The listing builds one solid part. Answer for the finished solid, in the listing's coordinates (mm). A direction names the side the tool comes from. Give positions to 0.01 mm unless a question says otherwise; leave off trailing zeros. Write each loop counter-clockwise with the first axis right and the second up, starting at its lowest first coordinate (ties: lowest second). Pieces come first, ordered by that corner, then holes. Notation, with made-up numbers: (-34.75, 68.5) - (20.25, 68.5) arc R22 cw to (20.25, 74.5) - close; hole circle Ø1 at (-7.75, 24.25). An arc over 180 degrees is marked (long way). Answer as CSV lines item,"result". Start each with the question number.
(1) Find section D-D (z = 14). Write down the section's boundary in (x, y), then the cut area to 3 significant figures.
(2) Find section A-A (z = 0). Write down the section's boundary in (x, y) (3 decimals).
(3) Find section C-C (z = 8.5). Write down the section's boundary in (x, y), then the cut area to 3 significant figures.
(4) Each of these flat-tipped pins is pushed along its axis until it touches: pin 1 Ø3.5 at (x, y) = (6.5, 5) entering from +Z; pin 2 Ø6 at (y, z) = (3.5, 9.5) entering from +X; pin 3 Ø5 at (y, z) = (-0.5, 12) entering from -X. Where does it stop, or does it pass through?
(5) Find section B-B (x = 32). Write down the section's boundary in (y, z), then the cut area to 3 significant figures.
(6) For faces 4 (the face through (28, 6, 0)), 5 (the face through (7, 5, -0.59)), 6 (the face through (12.77, 1.01, 2.21)), determine the directions among +Z, -Z, +X, -X, +Y, -Y from which every point of the face is accessible in a straight line to the end or side of a thin tool.
(7) For a pull along Y with two mould halves and no side action, classify faces 1 (the face through (9.57, 5.248, 0.995)), 2 (the face through (12.12, -2, 0)), 3 (the face through (35.5, 3, -2)) as pulls with the +Y half, pulls with the -Y half, needs draft (parallel to the pull), parting line crosses it, or undercut.
(8) Straight lines are drawn through the part: probe 1 along Y at (x, z) = (0, 9); probe 2 along Z at (x, y) = (18, 4.5); probe 3 along X at (y, z) = (1.5, 4). For each, find the intervals that lie inside material, in ascending order.
from build123d import *

# Parameters (mm, degrees)
BOSS_EXTRUDE3_DEPTH  = 3
SKETCH2_R            = 2.9999999999999982
BOSS_EXTRUDE4_DEPTH  = 16.205
SKETCH5_R            = 1.96
CUT_EXTRUDE2_DEPTH   = 32.80000000000002
SKETCH6_R            = 1.465
BOSS_EXTRUDE7_DEPTH  = 3
FILLET1_R            = 0.5
BOSS_EXTRUDE8_DEPTH  = 0.59
BOSS_EXTRUDE9_DEPTH  = 13.35
FILLET7_R            = 0.5
FILLET8_R            = 0.5
BOSS_EXTRUDE10_DEPTH = 3
CUT_EXTRUDE4_DEPTH   = 3
BOSS_EXTRUDE11_DEPTH = 0.59
BOSS_EXTRUDE12_DEPTH = 1.395
CUT_EXTRUDE6_DEPTH   = 20.895000000000014
CUT_EXTRUDE7_DEPTH   = 0.25
CUT_EXTRUDE8_DEPTH   = 0.25
FILLET9_R            = 0.5
FILLET10_R           = 0.5
CUT_EXTRUDE9_DEPTH   = 2.5
CUT_EXTRUDE10_DEPTH  = 2.5
CUT_EXTRUDE12_DEPTH  = 2.5
CUT_EXTRUDE14_START  = -2.5
CUT_EXTRUDE14_DEPTH  = 2.5


with BuildPart() as part:
    # Sketch1 → Boss-Extrude3 (new, symmetric)
    with BuildSketch(Plane.XY):
        with BuildLine():
            ThreePointArc((2.9999999999999982, 2.9999999999999973), (2.1213203435596406, 0.8786796564403563), (-5.5e-16, 0))
            Line((0, 0), (36.5, 0))
            Line((36.5, 0), (36.5, 6))
            Line((36.5, 6), (20.749999999999996, 5.999999999999999))
            ThreePointArc((20.749999999999996, 5.999999999999999), (20.435386233554034, 4.445031090493969), (19.54103584523481, 3.134669493650969))
            ThreePointArc((19.54103584523481, 3.1346694936509705), (17.593985916344508, 2.2872332130112563), (15.573673818645423, 2.9410609450836516))
            Line((15.573673818645423, 2.9410609450836516), (11.749999999999998, 5.9999999999999964))
            Line((11.749999999999998, 5.9999999999999964), (0, 5.9999999999999964))
            ThreePointArc((1.8e-16, 5.9999999999999964), (2.1213203435596415, 5.121320343559639), (2.9999999999999982, 2.9999999999999982))
        make_face()
    extrude(amount=BOSS_EXTRUDE3_DEPTH, both=True)

    # Sketch2 → Boss-Extrude4 (add, symmetric)
    with BuildSketch(Plane.XY):
        with Locations((0, 2.9999999999999982)):
            Circle(SKETCH2_R)
    extrude(amount=BOSS_EXTRUDE4_DEPTH, both=True)

    # Sketch5 → Cut-Extrude2 (cut)
    with BuildSketch(Plane.XY.offset(16.205)):
        with Locations((0, 2.9999999999999982)):
            Circle(SKETCH5_R)
    extrude(amount=-CUT_EXTRUDE2_DEPTH, mode=Mode.SUBTRACT)

    # Sketch6 → Boss-Extrude7 (add)
    with BuildSketch(Plane(origin=(36.5, 0, 0), x_dir=(0, 0, -1), z_dir=(1, 0, 0))):
        with Locations((0, 2.999999999999999)):
            Circle(SKETCH6_R)
    extrude(amount=BOSS_EXTRUDE7_DEPTH)

    # Fillet1
    fillet1_edges = [part.edges().sort_by_distance(p)[0] for p in [
        (39.5, 2.9999999999999987, 1.465),
    ]]
    fillet(fillet1_edges, radius=FILLET1_R)

    # Sketch12 → Boss-Extrude8 (add, symmetric)
    with BuildSketch(Plane.XY):
        with BuildLine():
            Line((12.12, -2.99e-15), (12.12, -3.970000000000003))
            Line((12.12, -3.970000000000003), (10.479512267647207, -5.6104877323527935))
            Line((10.479512267647207, -5.6104877323527935), (1.2595122676472073, -5.610487732352795))
            Line((1.2595122676472073, -5.610487732352795), (-2.8063517241754403, -1.5446237405301462))
            Line((-2.8063517241754403, -1.5446237405301462), (-2.8063517241754403, 1.939627423865778))
            ThreePointArc((-2.8063517241754403, 1.939627423865778), (-1.7057083970593148, 0.5320942351456543), (0, 0))
            Line((0, 0), (12.12, -2.99e-15))
        make_face()
    extrude(amount=BOSS_EXTRUDE8_DEPTH, both=True)

    # Sketch14 → Boss-Extrude9 (add, symmetric)
    with BuildSketch(Plane.XY):
        with BuildLine():
            Line((3.9999999999999982, 2.4999999999999982), (3.9999999999999982, 3.4999999999999982))
            Line((3.9999999999999982, 3.4999999999999982), (2.9580398915498067, 3.4999999999999982))
            ThreePointArc((2.9580398915498067, 3.4999999999999982), (2.999999999999999, 2.9999999999999982), (2.9580398915498067, 2.4999999999999982))
            Line((2.9580398915498067, 2.4999999999999982), (3.9999999999999982, 2.4999999999999982))
        make_face()
    extrude(amount=BOSS_EXTRUDE9_DEPTH, both=True)

    # Fillet7
    fillet7_edges = [part.edges().sort_by_distance(p)[0] for p in [
        (3.9999999999999982, 2.9999999999999982, 13.35),
    ]]
    fillet(fillet7_edges, radius=FILLET7_R)

    # Fillet8
    fillet8_edges = [part.edges().sort_by_distance(p)[0] for p in [
        (3.9999999999999982, 2.9999999999999982, -13.35),
    ]]
    fillet(fillet8_edges, radius=FILLET8_R)

    # Sketch15 → Boss-Extrude10 (add, symmetric)
    with BuildSketch(Plane.XY):
        Polygon((5.875, 5.9999999999999964), (27.07720850874597, 5.999999999999999), (27.07720850874597, 1.48970114733157), (5.875, 1.48970114733157), align=None)
    extrude(amount=BOSS_EXTRUDE10_DEPTH, both=True)

    # Sketch16 → Cut-Extrude4 (cut, symmetric)
    with BuildSketch(Plane.XY):
        with BuildLine():
            ThreePointArc((13.27019347571673, 1.2228284271177183), (12.760871493283885, 1.00722209344764), (12.214852275986694, 1.0953015306060352))
            Line((12.214852275986694, 1.0953015306060352), (1.8, 6))
            Line((1.8, 6), (19.169999999999998, 6.000000000000002))
            Line((19.169999999999998, 6.000000000000002), (13.27019347571673, 1.2228284271177183))
        make_face()
    extrude(amount=CUT_EXTRUDE4_DEPTH, both=True, mode=Mode.SUBTRACT)

    # Sketch17 → Boss-Extrude11 (add, symmetric)
    with BuildSketch(Plane.XY):
        Polygon((1.8, 6), (19.169999999999998, 5.999999999999999), (19.169999999999998, 0.49690997030879536), (1.8, 0.49690997030879536), (4.890483943976141, 2.396162656787146), align=None)
    extrude(amount=BOSS_EXTRUDE11_DEPTH, both=True)

    # Sketch19 → Boss-Extrude12 (add, symmetric)
    with BuildSketch(Plane.XY):
        with BuildLine():
            Line((8.17, 3.000156274700533), (10.684653005804094, 7.569117176028711))
            ThreePointArc((10.684653005804094, 7.569117176028711), (12.655773390851454, 8.734228825048191), (14.626946759842125, 7.569206818212221))
            Line((14.626946759842125, 7.569206818212221), (15.490695774172368, 5.999999999999999))
            Line((15.490695774172368, 5.999999999999999), (16.624997623308392, 3.9392692019970994))
            Line((16.624997623308392, 3.9392692019970994), (13.27019347571673, 1.2228284271177192))
            ThreePointArc((13.27019347571673, 1.2228284271177192), (12.760871493283883, 1.0072220934476446), (12.21485227598669, 1.0953015306060374))
            Line((12.21485227598669, 1.0953015306060374), (8.17, 3.000156274700533))
        make_face()
    extrude(amount=BOSS_EXTRUDE12_DEPTH, both=True)

    # Sketch20 → Cut-Extrude6 (cut, symmetric)
    with BuildSketch(Plane.XY.offset(1.395)):
        with BuildLine():
            ThreePointArc((14.155824552668768, 6.484228825629862), (12.655824552668768, 7.984228825629863), (11.155824552668768, 6.484228825629862))
            ThreePointArc((11.15582455266877, 6.484228825629865), (12.655824552668765, 4.984228825629861), (14.155824552668767, 6.484228825629859))
        make_face()
    extrude(amount=CUT_EXTRUDE6_DEPTH, both=True, mode=Mode.SUBTRACT)

    # Sketch21 → Cut-Extrude7 (cut, symmetric)
    with BuildSketch(Plane.XY.offset(1.395)):
        with BuildLine():
            Line((11.155824552668768, 6.484228825629862), (9.018377782257767, 2.60062711193924))
            Line((9.018377782257767, 2.60062711193924), (8.17, 3.000156274700535))
            Line((8.17, 3.000156274700535), (10.684653005804092, 7.569117176028711))
            ThreePointArc((10.684653005804092, 7.569117176028711), (12.655773390851452, 8.734228825048183), (14.626946759842125, 7.569206818212221))
            Line((14.626946759842125, 7.569206818212221), (16.62499762330839, 3.9392692019970985))
            Line((16.62499762330839, 3.9392692019970985), (15.886023032964967, 3.3409091724705715))
            Line((15.886023032964967, 3.3409091724705715), (14.155824552668767, 6.484228825629862))
            ThreePointArc((14.155824552668767, 6.484228825629862), (12.655824552668768, 4.984228825629862), (11.155824552668768, 6.484228825629862))
        make_face()
    extrude(amount=CUT_EXTRUDE7_DEPTH, both=True, mode=Mode.SUBTRACT)

    # Sketch22 → Cut-Extrude8 (cut, symmetric)
    with BuildSketch(Plane(origin=(0, 0, -1.395), x_dir=(-1, 0, 0), z_dir=(0, 0, -1))):
        with BuildLine():
            Line((-14.155824552668767, 6.484228825629862), (-15.886023032964967, 3.340909172470571))
            Line((-15.886023032964967, 3.340909172470571), (-16.624997623308392, 3.9392692019971034))
            Line((-16.624997623308392, 3.9392692019971034), (-14.626946759842125, 7.569206818212221))
            ThreePointArc((-14.626946759842125, 7.569206818212221), (-12.655773390851454, 8.73422882504819), (-10.684653005804092, 7.569117176028711))
            Line((-10.684653005804092, 7.569117176028711), (-8.17, 3.000156274700535))
            Line((-8.17, 3.000156274700535), (-9.018377782257769, 2.600627111939241))
            Line((-9.018377782257769, 2.600627111939241), (-11.155824552668768, 6.484228825629862))
            ThreePointArc((-11.155824552668768, 6.484228825629862), (-12.655824552668768, 4.984228825629864), (-14.155824552668767, 6.484228825629862))
        make_face()
    extrude(amount=CUT_EXTRUDE8_DEPTH, both=True, mode=Mode.SUBTRACT)

    # Fillet9
    fillet9_edges = [part.edges().sort_by_distance(p)[0] for p in [
        (15.625972191575258, 5.754238010104662, -1.145),
        (12.655773390851452, 8.73422882504819, -1.145),
        (9.427326502902046, 5.2846367253646225, -1.145),
    ]]
    fillet(fillet9_edges, radius=FILLET9_R)

    # Fillet10
    fillet10_edges = [part.edges().sort_by_distance(p)[0] for p in [
        (9.427326502902046, 5.2846367253646225, 1.145),
        (12.655773390851452, 8.734228825048183, 1.145),
        (15.625972191575258, 5.754238010104659, 1.145),
    ]]
    fillet(fillet10_edges, radius=FILLET10_R)

    # Sketch23 → Cut-Extrude9 (cut)
    with BuildSketch(Plane(origin=(0, 0, -3), x_dir=(-1, 0, 0), z_dir=(0, 0, -1))):
        Polygon((-35.5, 5), (-35.5, 1), (-14.230000308321648, 1), (-19.169999999999998, 5), align=None)
    extrude(amount=-CUT_EXTRUDE9_DEPTH, mode=Mode.SUBTRACT)

    # Sketch24 → Cut-Extrude10 (cut)
    with BuildSketch(Plane(origin=(0, 0, -3), x_dir=(-1, 0, 0), z_dir=(0, 0, -1))):
        with BuildLine():
            Line((-10.07009080824153, 1), (-3.4641016151377535, 1))
            ThreePointArc((-3.4641016151377535, 1), (-3.9566645904895195, 2.412798741174382), (-3.895636139676663, 3.9077549599121406))
            Line((-3.895636139676663, 3.9077549599121406), (-10.07009080824153, 1))
        make_face()
    extrude(amount=-CUT_EXTRUDE10_DEPTH, mode=Mode.SUBTRACT)

    # Sketch25 → Cut-Extrude12 (cut)
    with BuildSketch(Plane.XY.offset(3)):
        Polygon((19.524095671942906, 5), (35.5, 5), (35.5, 1), (14.584095980264548, 0.9999999999999983), align=None)
    extrude(amount=-CUT_EXTRUDE12_DEPTH, mode=Mode.SUBTRACT)

    # Sketch26 → Cut-Extrude14 (cut)
    with BuildSketch(Plane.XY.offset(3).offset(CUT_EXTRUDE14_START)):
        with BuildLine():
            Line((3.4641016151377535, 1), (10.070090808241538, 1))
            Line((10.070090808241538, 1), (3.8956361396766637, 3.9077549599121406))
            ThreePointArc((3.8956361396766637, 3.9077549599121406), (3.956664590489521, 2.4127987411743836), (3.4641016151377535, 1))
        make_face()
    extrude(amount=CUT_EXTRUDE14_DEPTH, mode=Mode.SUBTRACT)


solid = part.part
Result set:
1,outline,"circle Ø6 at (0, 3); hole circle Ø3.92 at (0, 3)"
1,area,"16.2 mm^2"
2,outline,"(-2.806, -1.545) - (1.26, -5.61) - (10.48, -5.61) - (12.12, -3.97) - (12.12, 0) - (36.5, 0) - (36.5, 1.535) - (39, 1.535) arc R0.5 ccw to (39.5, 2.035) - (39.5, 3.965) arc R0.5 ccw to (39, 4.465) - (36.5, 4.465) - (36.5, 6) - (15.491, 6) - (14.627, 7.569) arc R2.25 ccw to (10.685, 7.569) - (9.821, 6) - (0, 6) arc R3 ccw to (-2.806, 1.94) - close; hole circle Ø3.92 at (0, 3); hole circle Ø3 at (12.656, 6.484)"
3,outline,"(2.96, 2.5) - (4, 2.5) - (4, 3.5) - (2.96, 3.5) arc R3 ccw (long way) to start; hole circle Ø3.92 at (0, 3)"
3,area,"17.2 mm^2"
4,pin 1,"z = 3"
4,pin 2,"x = 4"
4,pin 3,"x = -2.83"
5,outline,"(0, -3) - (1, -3) - (1, -0.5) - (5, -0.5) - (5, -3) - (6, -3) - (6, 3) - (5, 3) - (5, 0.5) - (1, 0.5) - (1, 3) - (0, 3) - close"
5,area,"16.0 mm^2"
6,face 4,"+Z, -Z, +X, +Y"
6,face 5,"-Z, +Y"
6,face 6,"+Z, +Y"
7,face 1,"pulls with the +Y half"
7,face 2,"needs draft"
7,face 3,"undercut"
8,probe 1,"0 to 1.04, 4.96 to 6"
8,probe 2,"-3 to 3"
8,probe 3,"-2.6 to -1.26, 1.26 to 2.6"
